```python
from build123d import *

# Parameters (mm, degrees)
F1_DEPTH = 80
F2_R     = 2
F4_DEPTH = 25


with BuildPart() as f1:
    # F0 (on Top) → F1 (new body)
    with BuildSketch(Plane.XY):
        Polygon((25.391311, 40), (0, 40), (-25.391311, 40), (-40, 25.391311), (-40, 0), (-40, -25.391311), (-25.391311, -40), (0, -40), (25.391311, -40), (40, -25.391311), (40, 0), (40, 25.391311), align=None)
    extrude(amount=F1_DEPTH)

    # F2
    f2_edges = [f1.edges().sort_by_distance(p)[0] for p in [
        (32.695656, 32.695656, 80),
        (0, 40, 80),
        (-32.695656, 32.695656, 80),
        (-40, 0, 80),
        (-32.695656, -32.695656, 80),
        (0, -40, 80),
        (32.695656, -32.695656, 80),
        (40, 0, 80),
    ]]
    fillet(f2_edges, radius=F2_R)

    # F3 (on face) → F4 (cut)
    with BuildSketch(Plane.XY.offset(80)):
        with BuildLine():
            ThreePointArc((-8.873674, -17.226376), (0.143915, -11.989261), (9.009154, -17.480326))
            Line((9.009154, -17.480326), (0, 0))
            Line((0, 0), (-8.873674, -17.226376))
        make_face()
        with BuildLine():
            ThreePointArc((-8.873674, -17.226376), (-2.528532, -31.938364), (10.135299, -22.123538))
            ThreePointArc((10.135299, -22.123538), (9.84974, -19.734625), (9.009154, -17.480326))
            ThreePointArc((9.009154, -17.480326), (0.143915, -11.989261), (-8.873674, -17.226376))
        make_face()
    extrude(amount=-F4_DEPTH, mode=Mode.SUBTRACT)


solid = f1.part
```
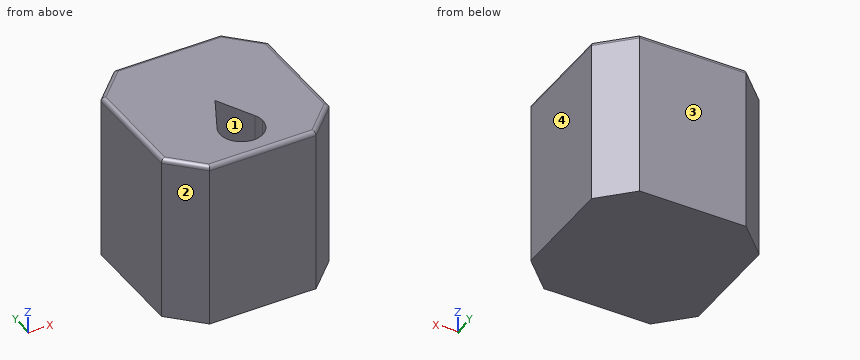
Geometry check sheet. Reference: the model listing, model coordinates, mm. Face numbers are marked on the shaded views. Round coordinates to 2 decimals unless told otherwise and drop trailing zeros. Write each loop counter-clockwise with the first axis right and the second up, starting at its lowest first coordinate (ties: lowest second). Pieces come first, ordered by that corner, then holes. Notation, with made-up numbers: (-3, 2) -> (7, 2) arc R31 cw to (7, 40) -> close; hole circle Ø10 at (-31.75, 12.25). An arc over 180 degrees is marked (long way). Put each result on its own line as item: value.
1) Cross-section at A-A, the plane z = 57. Enter the section's corners in (x, y).
Recorded:
outline: (-40, -25.39) -> (-25.39, -40) -> (25.39, -40) -> (40, -25.39) -> (40, 25.39) -> (25.39, 40) -> (-25.39, 40) -> (-40, 25.39) -> close; hole (-8.87, -17.23) arc R10.14 ccw (long way) to (10.14, -22.12) arc R10.14 ccw to (9.01, -17.48) -> (0, 0) -> close
2) Release check for a two-part mould opening along Y. For the marked faces 1, 2, 3 and 4 record: pulls with the +Y half, pulls with the -Y half, needs draft (parallel to the pull), parting line crosses it, or undercut.
Recorded:
face 1: undercut
face 2: pulls with the -Y half
face 3: pulls with the +Y half
face 4: needs draft
3) Cross-section at D-D, the plane y = -9.5. Enter the section's corners in (x, z).
Recorded:
outline: (-40, 0) -> (40, 0) -> (40, 78) arc R2 ccw to (38, 80) -> (4.9, 80) -> (4.9, 55) -> (-4.89, 55) -> (-4.89, 80) -> (-38, 80) arc R2 ccw to (-40, 78) -> close
4) Cross-section at C-C, the plane x = -3. Enter the section's corners in (y, z), plus the area to 3 significant figures.
Recorded:
outline: (-40, 0) -> (40, 0) -> (40, 78) arc R2 ccw to (38, 80) -> (-5.82, 80) -> (-5.82, 55) -> (-31.8, 55) -> (-31.8, 80) -> (-38, 80) arc R2 ccw to (-40, 78) -> close
area: 5,750 mm2
5) Thickness scan on probe 1 along X at (y, z) = (-22, 66.5); probe 2 along X at (y, z) = (-16.5, 72.5); probe 3 along Z at (x, y) = (3.5, -16.5). Record the ranges inside material, lowest first. Write a range as from..to.
Recorded:
probe 1: x = -40..-10.13, 10.13..40
probe 2: x = -40..-8.5, 8.5..40
probe 3: z = 0..55
6) Depth check by flat-ended pin: P1, Ø10, axis at x = 4.5, y = -23, coming from the +Z side; P2, Ø6, axis at x = -30, z = 58, coming from the +Y side; P3, Ø1, axis at x = -29, z = 55, coming from the +Y side. Enter the tip coordinate at first touch or a pass-through.
Recorded:
P1: stops at z = 55
P2: stops at y = 38.39
P3: stops at y = 36.89
7) Cross-section at B-B, the plane z = 24.5. Enter the section's corners in (x, y).
Recorded:
outline: (-40, -25.39) -> (-25.39, -40) -> (25.39, -40) -> (40, -25.39) -> (40, 25.39) -> (25.39, 40) -> (-25.39, 40) -> (-40, 25.39) -> close
